from build123d import *

# Parameters (mm, degrees)
SKETCH1_W           = 514.35
SKETCH1_H           = 76.2
SKETCH1_W_2         = 504.19
SKETCH1_H_2         = 66.04
BOSS_EXTRUDE1_DEPTH = 76.2
REVOLVE1_ANGLE      = 5
SKETCH3_W           = 38.1
SKETCH3_H           = 15.24
BOSS_EXTRUDE2_DEPTH = 5.08
SKETCH4_W           = 514.35
SKETCH4_H           = 76.2
BOSS_EXTRUDE3_DEPTH = 3.175


with BuildPart() as part:
    # Sketch1 → Boss-Extrude1 (new body)
    with BuildSketch(Plane(origin=(0, 0, 0), x_dir=(1, 0, 0), z_dir=(0, 1, 0))):
        Rectangle(SKETCH1_W, SKETCH1_H)
        Rectangle(SKETCH1_W_2, SKETCH1_H_2, mode=Mode.SUBTRACT)
    extrude(amount=BOSS_EXTRUDE1_DEPTH)

    # Sketch2 → Revolve1 (revolve)
    with BuildSketch(Plane(origin=(0, 0, -33.02), x_dir=(-1, 0, 0), z_dir=(0, 0, -1))):
        Polygon((-219.075, 12.7), (-219.075, 101.6), (-160.655, 101.6), (-160.655, 12.7), (-170.815, 12.7), (-170.815, 91.44), (-208.915, 91.44), (-208.915, 12.7), align=None)
        Polygon((-82.338333333, 12.7), (-92.498333333, 12.7), (-92.498333333, 101.6), (-34.078333333, 101.6), (-34.078333333, 12.7), (-44.238333333, 12.7), (-44.238333333, 91.44), (-82.338333333, 91.44), align=None)
        Polygon((44.238333333, 12.7), (34.078333333, 12.7), (34.078333333, 101.6), (92.498333333, 101.6), (92.498333333, 12.7), (82.338333333, 12.7), (82.338333333, 91.44), (44.238333333, 91.44), align=None)
        Polygon((170.815, 12.7), (160.655, 12.7), (160.655, 101.6), (219.075, 101.6), (219.075, 12.7), (208.915, 12.7), (208.915, 91.44), (170.815, 91.44), align=None)
    revolve(axis=Axis((275.97212821, -50.8, -33.02), (-1, 0, 0)), revolution_arc=REVOLVE1_ANGLE)

    # Sketch3 → Boss-Extrude2 (add)
    with BuildSketch(Plane.XY.offset(-33.02)):
        with Locations((-189.865, 83.82)):
            Rectangle(SKETCH3_W, SKETCH3_H)
        with Locations((-63.288333333, 83.82)):
            Rectangle(SKETCH3_W, SKETCH3_H)
        with Locations((63.288333333, 83.82)):
            Rectangle(SKETCH3_W, SKETCH3_H)
        with Locations((189.865, 83.82)):
            Rectangle(SKETCH3_W, SKETCH3_H)
    extrude(amount=-BOSS_EXTRUDE2_DEPTH)

    # Sketch4 → Boss-Extrude3 (add)
    with BuildSketch(Plane.XZ):
        Rectangle(SKETCH4_W, SKETCH4_H)
    extrude(amount=BOSS_EXTRUDE3_DEPTH)


solid = part.part
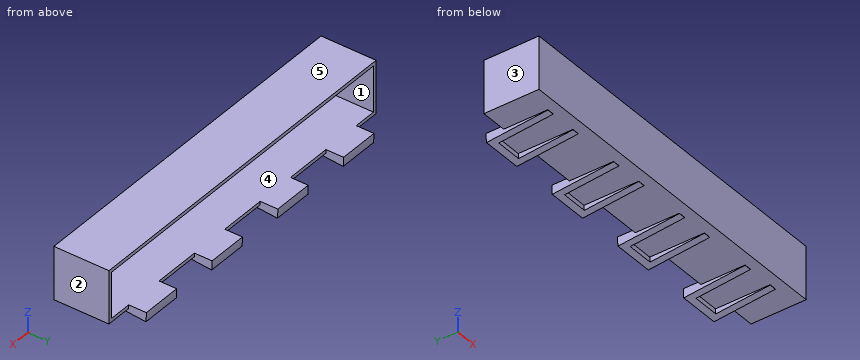
Could you check a few things on this model? Use its own coordinates, in mm. Face numbers are marked on the shaded views. A direction names the side the tool comes from. Give positions to 0.01 mm unless a question says otherwise; leave off trailing zeros. Order: outer loops, then holes, each group sorted by start corner. A loop starts at its lowest first (then second) coordinate and runs counter-clockwise, first axis right, second up. Notation, with made-up numbers: M -19.75,73.5 L 19.25,73.5 A27 cw 19.25,94.5 Z; hole C 26.25,-21.75 d11. An arc over 180 degrees is marked long. One line per question, with ' | ' between items.
1. We'd pull the mould along X, two halves only. Please class the marked faces 3, 4 and 5: +X half, -X half, draft (parallel to the pull), parting line (faces both ways), or undercut.
Results:
face 3: -X half | face 4: undercut | face 5: draft
2. For the marked faces 1 and 2, which set-ups out of +Z, -Z, +X, -X, +Y, -Y let a thin tool reach every point of the face, with its end or its side?
Results:
face 1: +Y | face 2: +Z, -Z, +X, +Y, -Y
3. I want a section at D-D (x = -180). List the corners of the cut face in (y, z) for me (3 decimals).
Results:
outline: M -3.175,-38.1 L 91.349,-38.1 A142.24 cw 90.899,-45.417 L 101.02,-46.303 A152.4 ccw 101.6,-33.02 L 0,-33.02 L 0,33.02 L 76.2,33.02 L 76.2,38.1 L -3.175,38.1 Z
4. If I drill on line 1 (X direction, y = 2, z = -1) (3 decimals); line 2 (Z direction, x = -130, y = 55.5); line 3 (Y direction, x = -122.5, z = -8.5) (3 decimals), over which ranges is the centre line in solid material (lowest first)?
Results:
line 1: -257.175 to -252.095, 252.095 to 257.175 | line 2: -38.1 to -33.02, 33.02 to 38.1 | line 3: -3.175 to 0
5. I want a section at A-A (x = 115.5). List the corners of the cut face in (y, z) for me (3 decimals), and give its area (3 significant figures).
Results:
outline: M -3.175,-38.1 L 76.2,-38.1 L 76.2,-33.02 L 0,-33.02 L 0,33.02 L 76.2,33.02 L 76.2,38.1 L -3.175,38.1 Z | area: 1,020 mm²
6. I'm going to push flat-ended pins straight in: pin 1 (8 mm diameter, centred on y = 43, z = -40, fed in from +X) (3 decimals); pin 2 (5.5 mm diameter, centred on x = -139.5, z = -35, fed in from +Y); pin 3 (5 mm diameter, centred on y = 82.5, z = -37.5, fed in from -X) (3 decimals); pin 4 (23 mm diameter, centred on x = -108, y = 39, fed in from -Z). Where does each tip first touch, or does it pass through?
Results:
pin 1: x = 257.175 | pin 2: y = 76.2 | pin 3: x = -219.075 | pin 4: z = -38.1
7. I want a section at C-C (z = 12.5). List the corners of the cut face in (x, y) for me (3 decimals), and give its area (3 significant figures).
Results:
outline: M -257.175,-3.175 L 257.175,-3.175 L 257.175,76.2 L 252.095,76.2 L 252.095,0 L -252.095,0 L -252.095,76.2 L -257.175,76.2 Z | area: 2,410 mm²
8. I want a section at B-B (y = 84). Give the number of separate pieces and of enclosed holes in the cut face, and give its area (3 significant figures).
Results:
separate pieces: 4 | enclosed holes: 0 | area: 1,730 mm²
